Design review of the part built by this model. Coordinates are the model's own, in mm. Face numbers are marked on the shaded views. A direction names the side the tool comes from. Coordinates: 2 decimals unless noted, no trailing zeros. Order: outer loops, then holes, each group sorted by start corner. A loop starts at its lowest first (then second) coordinate and runs counter-clockwise, first axis right, second up. Notation, with made-up numbers: M 58.5,0 L 110.5,0 A34 ccw 110.5,39 Z; hole C 71,-0.5 d9. An arc over 180 degrees is marked long. Answer in a Markdown table with one row per item.
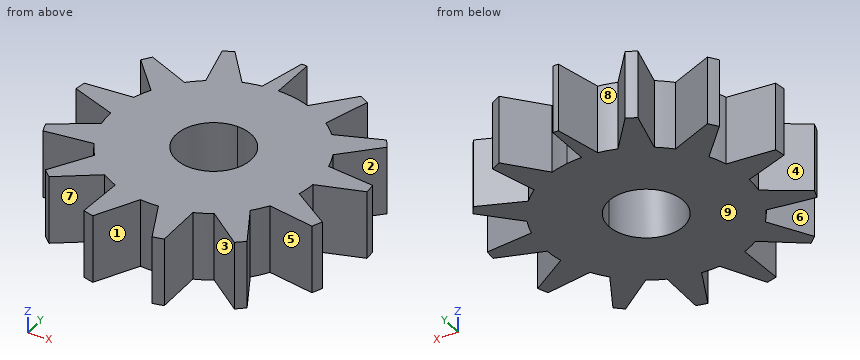
from build123d import *

# Parameters (mm, degrees)
BOSS_EXTRUDE1_DEPTH = 10


with BuildPart() as part:
    # Sketch1 → Boss-Extrude1 (new body)
    with BuildSketch(Plane.XY):
        with BuildLine():
            Line((0, 15), (0, 21.65))
            ThreePointArc((0, 21.65), (-0.40286299, 21.64625144), (-0.805586474, 21.635007059))
            Line((-0.805586474, 21.635007059), (-2.277654316, 14.826067949))
            ThreePointArc((-2.277654316, 14.826067949), (-3.589734964, 14.564127261), (-4.873254588, 14.18630994))
            Line((-4.873254588, 14.18630994), (-9.34097771, 19.531222067))
            ThreePointArc((-9.34097771, 19.531222067), (-10.061256675, 19.170122955), (-10.767600505, 18.782472664))
            Line((-10.767600505, 18.782472664), (-8.906780064, 12.069352464))
            ThreePointArc((-8.906780064, 12.069352464), (-9.946839874, 11.227661223), (-10.907759595, 10.296639288))
            Line((-10.907759595, 10.296639288), (-17.347636471, 12.953069476))
            ThreePointArc((-17.347636471, 12.953069476), (-17.817600697, 12.298601767), (-18.262887024, 11.627100134))
            Line((-18.262887024, 11.627100134), (-13.495469838, 6.547693781))
            ThreePointArc((-13.495469838, 6.547693781), (-14.02524364, 5.319073306), (-14.443428331, 4.048132663))
            Line((-14.443428331, 4.048132663), (-21.380160779, 3.40752477))
            ThreePointArc((-21.380160779, 3.40752477), (-21.492147124, 2.609619128), (-21.574366218, 1.808099086))
            Line((-21.574366218, 1.808099086), (-14.992510111, -0.473962639))
            ThreePointArc((-14.992510111, -0.473962639), (-14.890633111, -1.808050204), (-14.670281698, -3.12775237))
            Line((-14.670281698, -3.12775237), (-20.514747911, -6.918642796))
            ThreePointArc((-20.514747911, -6.918642796), (-20.243101654, -7.677195804), (-19.94341811, -8.425115673))
            Line((-19.94341811, -8.425115673), (-13.054946996, -7.38703993))
            ThreePointArc((-13.054946996, -7.38703993), (-12.344757988, -8.520971201), (-11.536350325, -9.587107028))
            Line((-11.536350325, -9.587107028), (-14.949653526, -15.659832676))
            ThreePointArc((-14.949653526, -15.659832676), (-14.356605551, -16.205257698), (-13.743673257, -16.728237964))
            Line((-13.743673257, -16.728237964), (-8.126652854, -12.607835397))
            ThreePointArc((-8.126652854, -12.607835397), (-6.970847581, -13.281840385), (-5.75958012, -13.850171004))
            Line((-5.75958012, -13.850171004), (-5.959773682, -20.813543611))
            ThreePointArc((-5.959773682, -20.813543611), (-5.181184132, -21.020890347), (-4.395418491, -21.199122536))
            Line((-4.395418491, -21.199122536), (-1.336640479, -14.940327715))
            ThreePointArc((-1.336640479, -14.940327715), (0, -15), (1.336640479, -14.940327715))
            Line((1.336640479, -14.940327715), (4.395418491, -21.199122536))
            ThreePointArc((4.395418491, -21.199122536), (5.181184132, -21.020890347), (5.959773682, -20.813543611))
            Line((5.959773682, -20.813543611), (5.75958012, -13.850171004))
            ThreePointArc((5.75958012, -13.850171004), (6.970847581, -13.281840385), (8.126652854, -12.607835397))
            Line((8.126652854, -12.607835397), (13.743673257, -16.728237964))
            ThreePointArc((13.743673257, -16.728237964), (14.356605551, -16.205257698), (14.949653526, -15.659832676))
            Line((14.949653526, -15.659832676), (11.536350325, -9.587107028))
            ThreePointArc((11.536350325, -9.587107028), (12.344757988, -8.520971201), (13.054946996, -7.38703993))
            Line((13.054946996, -7.38703993), (19.94341811, -8.425115673))
            ThreePointArc((19.94341811, -8.425115673), (20.243101654, -7.677195804), (20.514747911, -6.918642796))
            Line((20.514747911, -6.918642796), (14.670281698, -3.12775237))
            ThreePointArc((14.670281698, -3.12775237), (14.890633111, -1.808050204), (14.992510111, -0.473962639))
            Line((14.992510111, -0.473962639), (21.574366218, 1.808099086))
            ThreePointArc((21.574366218, 1.808099086), (21.492147124, 2.609619128), (21.380160779, 3.40752477))
            Line((21.380160779, 3.40752477), (14.443428331, 4.048132663))
            ThreePointArc((14.443428331, 4.048132663), (14.02524364, 5.319073306), (13.495469838, 6.547693781))
            Line((13.495469838, 6.547693781), (18.262887024, 11.627100134))
            ThreePointArc((18.262887024, 11.627100134), (17.817600697, 12.298601767), (17.347636471, 12.953069476))
            Line((17.347636471, 12.953069476), (10.907759595, 10.296639288))
            ThreePointArc((10.907759595, 10.296639288), (9.946839874, 11.227661223), (8.906780064, 12.069352464))
            Line((8.906780064, 12.069352464), (10.767600505, 18.782472664))
            ThreePointArc((10.767600505, 18.782472664), (10.061256675, 19.170122955), (9.34097771, 19.531222067))
            Line((9.34097771, 19.531222067), (4.873254588, 14.18630994))
            ThreePointArc((4.873254588, 14.18630994), (3.589734964, 14.564127261), (2.277654316, 14.826067949))
            ThreePointArc((2.277654316, 14.826067949), (1.142142892, 14.956453778), (0, 15))
        make_face()
        with BuildLine():
            ThreePointArc((5.5, 0), (-3.889087297, -3.889087297), (0, 5.5))
            ThreePointArc((0, 5.5), (3.889087297, 3.889087297), (5.5, 0))
        make_face(mode=Mode.SUBTRACT)
    extrude(amount=BOSS_EXTRUDE1_DEPTH)


solid = part.part
(1) Insertion check: pin 1 Ø2 at (y, z) = (-3, 2.5) entering from -X; pin 2 Ø5 at (x, z) = (-10.5, 8) entering from -Y; pin 3 Ø3 at (x, z) = (8.5, 4.5) entering from +Y. Each pin has a flat end and moves straight along its axis. Give the tip position at first contact, or say it passes through.
Return value:
| item | result |
|---|---|
| pin 1 | stops at x = -16.02 |
| pin 2 | stops at y = -16.18 |
| pin 3 | stops at y = 19.53 |
(2) For the marked faces 5, 6, 7, 8 and 9, list the 3-axis set-ups (+Z, -Z, +X, -X, +Y, -Y) from which the entire face can be reached by the end or side of a thin tool; tool diameter is ignored.
Return value:
| item | result |
|---|---|
| face 5 | +Z, -Z |
| face 6 | +Z, -Z, -X |
| face 7 | +Z, -Z, -Y |
| face 8 | +Z, -Z, +Y |
| face 9 | -Z, +X, -X, +Y, -Y |
(3) Add section A-A, the plane y = 9.5. Give the boundary of the cut face in (x, z).
Return value:
| item | result |
|---|---|
| outline | M -16.27,0 L 16.27,0 L 16.27,10 L -16.27,10 Z |
(4) For line 1 along Y through (x, z) = (17, 1.5); line 2 along Y through (x, z) = (-18, 7.25); line 3 along X through (y, z) = (11.5, 0.75), list the stretches that pass through material, from the lowest coordinate up. Write a range as from..to.
Return value:
| item | result |
|---|---|
| line 1 | y = -7.98..-4.64, 0.22..3.81, 10.28..12.81 |
| line 2 | y = -8.13..-5.29, 0.57..3.72, 11.35..12.03 |
| line 3 | x = -18.14..-13.83, -9.63..9.63, 13.83..18.14 |
(5) Draft analysis for pull direction X (two halves, no side actions). For the marked faces 1, 2, 3 and 4, state which applies: pulls with the +X half, pulls with the -X half, needs draft (parallel to the pull), parting line crosses it, or undercut.
Return value:
| item | result |
|---|---|
| face 1 | undercut |
| face 2 | pulls with the +X half |
| face 3 | undercut |
| face 4 | pulls with the -X half |
